from build123d import *

# Parameters (mm, degrees)
SKETCH1_R           = 9.525
BOSS_EXTRUDE1_DEPTH = 7.9375
SKETCH2_R           = 7.62
BOSS_EXTRUDE2_DEPTH = 4.7625
SKETCH3_R           = 11.1125
BOSS_EXTRUDE3_DEPTH = 3.175
FILLET1_R           = 0.635
FILLET3_R           = 0.635
FILLET4_R           = 0.635


with BuildPart() as part:
    # Sketch1 → Boss-Extrude1 (new body)
    with BuildSketch(Plane(origin=(0, 0, 0), x_dir=(1, 0, 0), z_dir=(0, 1, 0))):
        with Locations(Location((0, 0, 0), (0, 0, 270))):
            Circle(SKETCH1_R)
        Polygon((5.865878735, 0), (2.932939367, 5.08), (-2.932939367, 5.08), (-5.865878735, 0), (-2.932939367, -5.08), (2.932939367, -5.08), align=None, mode=Mode.SUBTRACT)
    extrude(amount=BOSS_EXTRUDE1_DEPTH)

    # Sketch2 → Boss-Extrude2 (add)
    with BuildSketch(Plane(origin=(0, 7.9375, 0), x_dir=(1, 0, 0), z_dir=(0, 1, 0))):
        with Locations(Location((0, 0, 0), (0, 0, 90))):
            Circle(SKETCH2_R)
        Polygon((-2.932939367, 5.08), (-5.865878735, 0), (-2.932939367, -5.08), (2.932939367, -5.08), (5.865878735, 0), (2.932939367, 5.08), align=None, mode=Mode.SUBTRACT)
    extrude(amount=BOSS_EXTRUDE2_DEPTH)

    # Sketch3 → Boss-Extrude3 (add)
    with BuildSketch(Plane.XZ):
        with Locations(Location((0, 0, 0), (0, 0, 270))):
            Circle(SKETCH3_R)
        Polygon((-2.932939367, 5.08), (2.932939367, 5.08), (5.865878735, 0), (2.932939367, -5.08), (-2.932939367, -5.08), (-5.865878735, 0), align=None, mode=Mode.SUBTRACT)
    extrude(amount=BOSS_EXTRUDE3_DEPTH)

    # Fillet1
    fillet1_edges = [part.edges().sort_by_distance(p)[0] for p in [
        (0, 0, -9.525),
        (0, 0, 11.1125),
    ]]
    fillet(fillet1_edges, radius=FILLET1_R)

    # Fillet3
    fillet3_edges = [part.edges().sort_by_distance(p)[0] for p in [
        (0, 12.7, -5.08),
        (-4.399409051, 12.7, -2.54),
        (-4.399409051, 12.7, 2.54),
        (0, 12.7, 5.08),
        (4.399409051, 12.7, 2.54),
        (4.399409051, 12.7, -2.54),
    ]]
    fillet(fillet3_edges, radius=FILLET3_R)

    # Fillet4
    fillet4_edges = [part.edges().sort_by_distance(p)[0] for p in [
        (0, 12.7, 7.62),
        (0, 7.9375, 7.62),
        (0, 7.9375, -9.525),
    ]]
    fillet(fillet4_edges, radius=FILLET4_R)


solid = part.part
The model under review builds one solid part; all positions refer to its coordinate system, in mm. A direction names the side the tool comes from. Round coordinates to 2 decimals unless told otherwise and drop trailing zeros. Loops run counter-clockwise (first coordinate to the right, second up) from the corner with the lowest first, then second, coordinate; pieces in that order, holes last. Notation, with made-up numbers: M -17.75,29.5 L 16.25,29.5 A13 cw 16.25,53.5 Z; hole C 59.5,-15.75 d7. An arc over 180 degrees is marked long. Answer as CSV lines item,"result".
1. We need section B-B (y = 9.25). Give the boundary of the cut face in (x, z).
Outcome:
outline,"C 0,0 d15.24; hole M -5.87,0 L -2.93,-5.08 L 2.93,-5.08 L 5.87,0 L 2.93,5.08 L -2.93,5.08 Z"
2. We need section C-C (y = 5.75). Give the boundary of the cut face in (x, z) (3 decimals), plus the area to 3 significant figures.
Outcome:
outline,"C 0,0 d19.05; hole M -5.866,0 L -2.933,-5.08 L 2.933,-5.08 L 5.866,0 L 2.933,5.08 L -2.933,5.08 Z"
area,"196 mm2"
3. To check wall thickness, follow L1, parallel to Y at x = -9, z = -4.5 (3 decimals); L2, parallel to Z at x = 3.75, y = 11; L3, parallel to Z at x = -1.5, y = -2. State the ranges of each line that lie inside material, in increasing order. Write a range as [from, to].
Outcome:
L1,"y = [-3.175, 0.008]"
L2,"z = [-6.63, -3.66], [3.66, 6.63]"
L3,"z = [-11.01, -5.08], [5.08, 11.01]"
4. For faces 4 (the face through (-5, -3.175, -2)), 5 (the face through (-8, 7.938, 3)), 6 (the face through (0, 5, -5.08)), list the 3-axis set-ups (+Z, -Z, +X, -X, +Y, -Y) from which the entire face can be reached by the end or side of a thin tool; tool diameter is ignored.
Outcome:
face 4,"+Z, -Z, +X, -X, -Y"
face 5,"+Y"
face 6,"+Y, -Y"
5. Insertion check: pin 1 Ø3 at (x, y) = (1, 6.5) entering from -Z (3 decimals); pin 2 Ø1.5 at (x, y) = (4, 4.5) entering from +Z; pin 3 Ø4.5 at (x, y) = (1.5, 7.5) entering from +Z (3 decimals). Each pin has a flat end and moves straight along its axis. Give the tip position at first contact, or say it passes through.
Outcome:
pin 1,"stops at z = -9.525"
pin 2,"stops at z = 8.95"
pin 3,"stops at z = 9.525"
6. Draft analysis for pull direction X (two halves, no side actions). For faces 1 (the face through (-5.796, 3.922, -7.559)), 2 (the face through (0, 12.7, 6)), 3 (the face through (4.42, 4.552, -2.504)), state which applies: pulls with the +X half, pulls with the -X half, needs draft (parallel to the pull), parting line crosses it, or undercut.
Outcome:
face 1,"parting line crosses it"
face 2,"needs draft"
face 3,"undercut"
